Model file for the job. Use its own axes, mm. Face numbers are marked on the shaded views. A direction names the side the tool comes from. Round coordinates to 2 decimals unless told otherwise and drop trailing zeros. Loops run counter-clockwise (first coordinate to the right, second up) from the corner with the lowest first, then second, coordinate; pieces in that order, holes last. Notation, with made-up numbers: (78.5, 55.5) - (127.5, 55.5) arc R24 ccw to (127.5, 76.5) - close; hole circle Ø3 at (12, 41.25). An arc over 180 degrees is marked (long way). Answer as a JSON object with one key per item and string values.
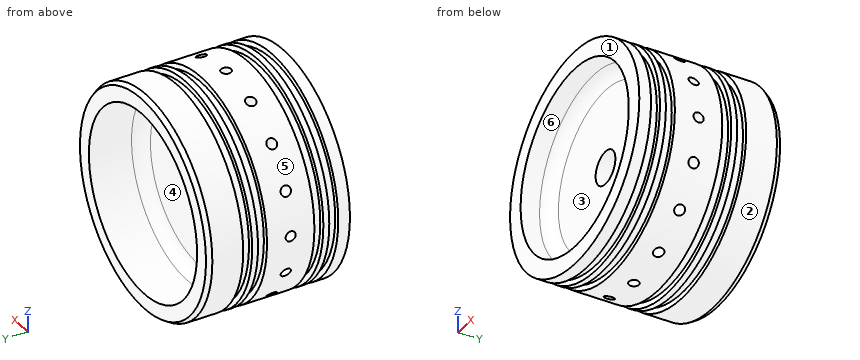
from build123d import *

# Parameters (mm, degrees)
HOLEPATTERN_COUNT             = 16
CHAMFER2_SIZE                 = 2.54
CHAMFER2_SIZE2                = 1.466469684
FILLET1_R                     = 6.35
PIPE_TAP_DRILL_FOR_1_2_TAP1_D = 17.8562


with BuildPart() as part:
    # Sketch1 → Revolve1 (revolve)
    with BuildSketch(Plane.XY):
        Polygon((0, -15.24), (0, 0), (-58.4581, 0), (-58.4581, -12.7), (-55.6641, -12.7), (-55.6641, -17.5006), (-58.4581, -17.5006), (-58.4581, -20.6756), (-55.6641, -20.6756), (-55.6641, -25.4762), (-58.4581, -25.4762), (-58.4581, -31.75), (-48.9331, -31.75), (-48.9331, -15.24), align=None)
        Polygon((-58.4581, 0), (0, 0), (0, 15.3162), (-48.9331, 15.3162), (-48.9331, 44.5262), (-58.4581, 44.5262), (-58.4581, 25.4762), (-55.6387, 25.4762), (-55.6387, 20.6756), (-58.4581, 20.6756), (-58.4581, 17.5006), (-55.6387, 17.5006), (-55.6387, 12.7), (-58.4581, 12.7), align=None)
    revolve(axis=Axis((0, 31.75, 0), (0, -1, 0)))

    # Sketch4 → Tap Drill for 1/4-28 Tap1 (revolve, cut)
    with BuildSketch(Plane(origin=(0, 0, 58.4581), x_dir=(0, -1, 0), z_dir=(1, 0, 0))):
        Polygon((0, 0), (0, 20.675388061), (2.7051, 19.05), (2.7051, 0), align=None)
    tap_drill_for_1_4_28_tap1 = revolve(axis=Axis((0, 0, 64.8081), (0, 0, -1)), mode=Mode.SUBTRACT)

    # HolePattern: Tap Drill for 1/4-28 Tap1 ×16 about axis
    holepattern_axis = Axis((0, -12.7, 0), (0, 1, 0))
    for i in range(1, HOLEPATTERN_COUNT):
        add(tap_drill_for_1_4_28_tap1.rotate(holepattern_axis, i * 360 / HOLEPATTERN_COUNT), mode=Mode.SUBTRACT)

    # Chamfer2
    chamfer2_edges = [part.edges().sort_by_distance(p)[0] for p in [
        (58.4581, 44.5262, 0),
    ]]
    chamfer2_side = [part.faces().sort_by_distance(p)[0] for p in [
        (58.4581, 35.0012, 0),
    ]]
    chamfer(chamfer2_edges, length=CHAMFER2_SIZE, length2=CHAMFER2_SIZE2, reference=chamfer2_side[0])

    # Fillet1
    fillet1_edges = [part.edges().sort_by_distance(p)[0] for p in [
        (48.9331, 15.3162, 0),
        (48.9331, -15.24, 0),
    ]]
    fillet(fillet1_edges, radius=FILLET1_R)

    # Pipe Tap Drill for 1/2 Tap1 (through all)
    with Locations(Plane(origin=(0, 15.3162, 0), x_dir=(1, 0, 0), z_dir=(0, 1, 0))):
        with Locations((0, 0)):
            Hole(PIPE_TAP_DRILL_FOR_1_2_TAP1_D / 2)


solid = part.part
1) Slice it at C-C on y = 27.5. List the corners of the cut face in (x, z).
Values follow:
{"outline": "circle Ø116.92 at (0, 0); hole circle Ø97.87 at (0, 0)"}
2) Slice it at A-A on y = 6. List the corners of the cut face in (x, z), then the cut area to 3 significant figures.
Values follow:
{"outline": "circle Ø116.92 at (0, 0); hole circle Ø17.86 at (0, 0)", "area": "10,500 mm²"}
3) Two-plate mould, pull along Z, no slides. Class the marked faces 1, 2 and 3: pulls with the +Z half, pulls with the -Z half, needs draft (parallel to the pull), parting line crosses it, or undercut.
Values follow:
{"face 1": "needs draft", "face 2": "parting line crosses it", "face 3": "undercut"}
4) Slice it at B-B on z = -46.5. Count the separate pieces of the cut face and the enclosed holes in it, then the cut area to 3 significant figures.
Values follow:
{"separate pieces": "1", "enclosed holes": "3", "area": "3,890 mm²"}
5) Probe probe 1 along X at (y, z) = (-28, 1.5); probe 2 along X at (y, z) = (26.5, 0). List the from-to ranges inside material, lowest first.
Values follow:
{"probe 1": "-58.44 to -48.91, 48.91 to 58.44", "probe 2": "-58.46 to -48.93, 48.93 to 58.46"}
6) Tool access for the marked faces 4, 5 and 6: list every direction of +Z, -Z, +X, -X, +Y, -Y with a clear straight run to the whole face (end or side of a thin tool).
Values follow:
{"face 4": "+Y", "face 5": "+Y, -Y", "face 6": "-Y"}
7) Drop flat-ended pins along their axis: P1, Ø4, axis at x = 23, y = -4.5, coming from the -Z side; P2, Ø1, axis at x = -33, y = 25.5, coming from the +Z side; P3, Ø3, axis at x = 0, y = 0, coming from the +Z side. Give the stop position or say it passes through.
Values follow:
{"P1": "z = -54.56", "P2": "z = 48.59", "P3": "z = 38.68"}
